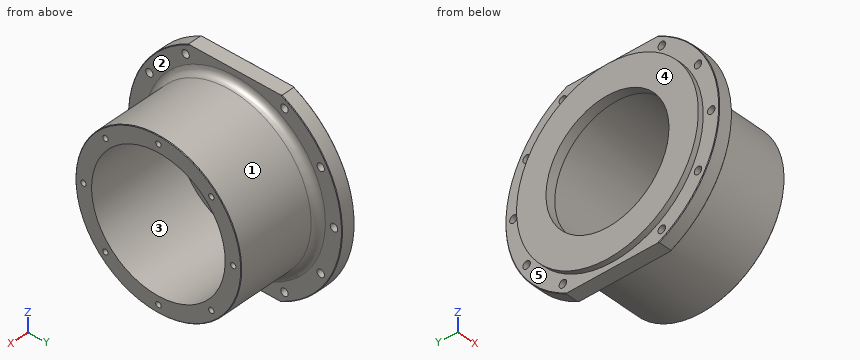
from build123d import *

# Parameters (mm, degrees)
CUT_EXTRUDE_1_REACH = 163.991
CUT_EXTRUDE_2_REACH = 164.985
SKETCH_5_R          = 3.5
SKETCH_6_R          = 2.5
CUT_EXTRUDE_3_DEPTH = 15
FILLET_1_R          = 7
CHAMFER_1_SIZE      = 0.5


with BuildPart() as part:
    # 草图1 → 旋转1 (revolve)
    with BuildSketch(Plane.XY, mode=Mode.PRIVATE) as revolve_1_sk:
        Polygon((0, 0), (0, 85), (5, 85), (5, 100), (18, 100), (18, 77.5), (97, 77.5), (97, 0), align=None)
    revolve(revolve_1_sk.sketch.rotate(Axis((0, 0, 0), (-1, 0, 0)), 90), axis=Axis((0, 0, 0), (-1, 0, 0)))

    # 草图3 → 切除-旋转1 (revolve, cut)
    with BuildSketch(Plane.XY, mode=Mode.PRIVATE) as cut_revolve_1_sk:
        Polygon((0, 0), (0, 57.5), (9, 57.5), (9, 62.5), (97, 62.5), (97, 0), align=None)
    revolve(cut_revolve_1_sk.sketch.rotate(Axis((97, 0, 0), (-1, 0, 0)), 90), axis=Axis((97, 0, 0), (-1, 0, 0)), mode=Mode.SUBTRACT)

    # 草图4 → 切除-拉伸1 (cut, up to next)
    with BuildSketch(Plane(origin=(18, 0, 0), x_dir=(0, 0, -1), z_dir=(1, 0, 0)), mode=Mode.PRIVATE) as cut_extrude_1_sk1:
        with BuildLine():
            Line((-90, 43.588989435), (-90, -43.588989435))
            ThreePointArc((-90, -43.588989435), (-100, 0), (-90, 43.588989435))
        make_face()
    cut_extrude_1_tool1 = extrude(cut_extrude_1_sk1.sketch, amount=-CUT_EXTRUDE_1_REACH, mode=Mode.PRIVATE) & part.part
    # 草图4 → 切除-拉伸1 (cut, up to next)
    with BuildSketch(Plane(origin=(18, 0, 0), x_dir=(0, 0, -1), z_dir=(1, 0, 0)), mode=Mode.PRIVATE) as cut_extrude_1_sk2:
        with BuildLine():
            Line((90, 43.588989435), (90, -43.588989435))
            ThreePointArc((90, -43.588989435), (100, 0), (90, 43.588989435))
        make_face()
    cut_extrude_1_tool2 = extrude(cut_extrude_1_sk2.sketch, amount=-CUT_EXTRUDE_1_REACH, mode=Mode.PRIVATE) & part.part
    add(cut_extrude_1_tool1.solids().sort_by_distance((18, 0, 94.017654))[0], mode=Mode.SUBTRACT)
    add(cut_extrude_1_tool2.solids().sort_by_distance((18, 0, -94.017654))[0], mode=Mode.SUBTRACT)

    # 草图5 → 切除-拉伸2 (cut, up to next)
    with BuildSketch(Plane.ZY.offset(-5), mode=Mode.PRIVATE) as cut_extrude_2_sk1:
        with Locations((0, 92.5)):
            Circle(SKETCH_5_R)
    cut_extrude_2_tool1 = extrude(cut_extrude_2_sk1.sketch, amount=-CUT_EXTRUDE_2_REACH, mode=Mode.PRIVATE) & part.part
    # 草图5 → 切除-拉伸2 (cut, up to next)
    with BuildSketch(Plane.ZY.offset(-5), mode=Mode.PRIVATE) as cut_extrude_2_sk2:
        with Locations((46.25, 80.10734985)):
            Circle(SKETCH_5_R)
    cut_extrude_2_tool2 = extrude(cut_extrude_2_sk2.sketch, amount=-CUT_EXTRUDE_2_REACH, mode=Mode.PRIVATE) & part.part
    # 草图5 → 切除-拉伸2 (cut, up to next)
    with BuildSketch(Plane.ZY.offset(-5), mode=Mode.PRIVATE) as cut_extrude_2_sk3:
        with Locations((80.10734985, 46.25)):
            Circle(SKETCH_5_R)
    cut_extrude_2_tool3 = extrude(cut_extrude_2_sk3.sketch, amount=-CUT_EXTRUDE_2_REACH, mode=Mode.PRIVATE) & part.part
    # 草图5 → 切除-拉伸2 (cut, up to next)
    with BuildSketch(Plane.ZY.offset(-5), mode=Mode.PRIVATE) as cut_extrude_2_sk4:
        with Locations((80.10734985, -46.25)):
            Circle(SKETCH_5_R)
    cut_extrude_2_tool4 = extrude(cut_extrude_2_sk4.sketch, amount=-CUT_EXTRUDE_2_REACH, mode=Mode.PRIVATE) & part.part
    # 草图5 → 切除-拉伸2 (cut, up to next)
    with BuildSketch(Plane.ZY.offset(-5), mode=Mode.PRIVATE) as cut_extrude_2_sk5:
        with Locations((46.25, -80.10734985)):
            Circle(SKETCH_5_R)
    cut_extrude_2_tool5 = extrude(cut_extrude_2_sk5.sketch, amount=-CUT_EXTRUDE_2_REACH, mode=Mode.PRIVATE) & part.part
    # 草图5 → 切除-拉伸2 (cut, up to next)
    with BuildSketch(Plane.ZY.offset(-5), mode=Mode.PRIVATE) as cut_extrude_2_sk6:
        with Locations((0, -92.5)):
            Circle(SKETCH_5_R)
    cut_extrude_2_tool6 = extrude(cut_extrude_2_sk6.sketch, amount=-CUT_EXTRUDE_2_REACH, mode=Mode.PRIVATE) & part.part
    # 草图5 → 切除-拉伸2 (cut, up to next)
    with BuildSketch(Plane.ZY.offset(-5), mode=Mode.PRIVATE) as cut_extrude_2_sk7:
        with Locations((-46.25, -80.10734985)):
            Circle(SKETCH_5_R)
    cut_extrude_2_tool7 = extrude(cut_extrude_2_sk7.sketch, amount=-CUT_EXTRUDE_2_REACH, mode=Mode.PRIVATE) & part.part
    # 草图5 → 切除-拉伸2 (cut, up to next)
    with BuildSketch(Plane.ZY.offset(-5), mode=Mode.PRIVATE) as cut_extrude_2_sk8:
        with Locations((-80.10734985, -46.25)):
            Circle(SKETCH_5_R)
    cut_extrude_2_tool8 = extrude(cut_extrude_2_sk8.sketch, amount=-CUT_EXTRUDE_2_REACH, mode=Mode.PRIVATE) & part.part
    # 草图5 → 切除-拉伸2 (cut, up to next)
    with BuildSketch(Plane.ZY.offset(-5), mode=Mode.PRIVATE) as cut_extrude_2_sk9:
        with Locations((-80.10734985, 46.25)):
            Circle(SKETCH_5_R)
    cut_extrude_2_tool9 = extrude(cut_extrude_2_sk9.sketch, amount=-CUT_EXTRUDE_2_REACH, mode=Mode.PRIVATE) & part.part
    # 草图5 → 切除-拉伸2 (cut, up to next)
    with BuildSketch(Plane.ZY.offset(-5), mode=Mode.PRIVATE) as cut_extrude_2_sk10:
        with Locations((-46.25, 80.10734985)):
            Circle(SKETCH_5_R)
    cut_extrude_2_tool10 = extrude(cut_extrude_2_sk10.sketch, amount=-CUT_EXTRUDE_2_REACH, mode=Mode.PRIVATE) & part.part
    add(cut_extrude_2_tool1.solids().sort_by_distance((5, 92.5, 0))[0], mode=Mode.SUBTRACT)
    add(cut_extrude_2_tool2.solids().sort_by_distance((5, 80.10735, 46.25))[0], mode=Mode.SUBTRACT)
    add(cut_extrude_2_tool3.solids().sort_by_distance((5, 46.25, 80.10735))[0], mode=Mode.SUBTRACT)
    add(cut_extrude_2_tool4.solids().sort_by_distance((5, -46.25, 80.10735))[0], mode=Mode.SUBTRACT)
    add(cut_extrude_2_tool5.solids().sort_by_distance((5, -80.10735, 46.25))[0], mode=Mode.SUBTRACT)
    add(cut_extrude_2_tool6.solids().sort_by_distance((5, -92.5, 0))[0], mode=Mode.SUBTRACT)
    add(cut_extrude_2_tool7.solids().sort_by_distance((5, -80.10735, -46.25))[0], mode=Mode.SUBTRACT)
    add(cut_extrude_2_tool8.solids().sort_by_distance((5, -46.25, -80.10735))[0], mode=Mode.SUBTRACT)
    add(cut_extrude_2_tool9.solids().sort_by_distance((5, 46.25, -80.10735))[0], mode=Mode.SUBTRACT)
    add(cut_extrude_2_tool10.solids().sort_by_distance((5, 80.10735, -46.25))[0], mode=Mode.SUBTRACT)

    # 草图6 → 切除-拉伸3 (cut)
    with BuildSketch(Plane(origin=(97, 0, 0), x_dir=(0, 0, -1), z_dir=(1, 0, 0))):
        with Locations((0, 70)):
            Circle(SKETCH_6_R)
        with Locations((49.497474683, 49.497474683)):
            Circle(SKETCH_6_R)
        with Locations((70, 0)):
            Circle(SKETCH_6_R)
        with Locations((49.497474683, -49.497474683)):
            Circle(SKETCH_6_R)
        with Locations((0, -70)):
            Circle(SKETCH_6_R)
        with Locations((-49.497474683, -49.497474683)):
            Circle(SKETCH_6_R)
        with Locations((-70, 0)):
            Circle(SKETCH_6_R)
        with Locations((-49.497474683, 49.497474683)):
            Circle(SKETCH_6_R)
    extrude(amount=-CUT_EXTRUDE_3_DEPTH, mode=Mode.SUBTRACT)

    # 圆角1
    fillet_1_edges = [part.edges().sort_by_distance(p)[0] for p in [
        (18, 0, 77.5),
    ]]
    fillet(fillet_1_edges, radius=FILLET_1_R)

    # 倒角1
    chamfer_1_edges = [part.edges().sort_by_distance(p)[0] for p in [
        (18, -100, 0),
        (5, -100, 0),
        (97, 0, 77.5),
        (18, 100, 0),
        (5, 100, 0),
    ]]
    chamfer(chamfer_1_edges, length=CHAMFER_1_SIZE)


solid = part.part
CAD build for the part. Positions are in the model's coordinates, mm. Face numbers are marked on the shaded views. A direction names the side the tool comes from. Coordinates: 2 decimals unless noted, no trailing zeros. Write each loop counter-clockwise with the first axis right and the second up, starting at its lowest first coordinate (ties: lowest second). Pieces come first, ordered by that corner, then holes. Notation, with made-up numbers: (-28, 29) - (-2, 29) arc R15 ccw to (-2, 49) - close; hole circle Ø11 at (-8.5, -13.5). An arc over 180 degrees is marked (long way). Use a Markdown table: item, result. Add a question column.
Item 1: Band-saw the part on B-B, the plane z = 0. Give the number of separate pieces and of enclosed holes in the cut face, and give its area (3 significant figures).
Item 2: Mould opens along Z. For the marked faces 1, 2 and 3 say: pulls with the +Z half, pulls with the -Z half, needs draft (parallel to the pull), parting line crosses it, or undercut.
Item 3: Band-saw the part on A-A, the plane x = 40.5. Give the cut face in (y, z).
Item 4: Drill centre lines: L1, parallel to Y at x = 14, z = 0; L2, parallel to Y at x = 90, z = 0; L3, parallel to Z at x = 10.5, y = -77. Where is each one in solid material? Low to high. Write a range as from..to.
Item 5: Flat gauge pins, fed straight in: pin 1 (4.5 mm diameter, centred on y = 49.5, z = 49.5, fed in from +X); pin 2 (1 mm diameter, centred on x = 26, z = 39.5, fed in from +Y); pin 3 (10 mm diameter, centred on x = 64.5, y = 34.5, fed in from -Z). Where does each tip first touch, or does it go through?
Item 6: 3-axis set-ups, long thin cutter, end or side, ignore diameter. For the marked faces 4 and 5: which of +Z, -Z, +X, -X, +Y, -Y reach the whole face in a straight line?
Numbers:
| question | item | result |
|---|---|---|
| 1 | separate pieces | 4 |
| 1 | enclosed holes | 0 |
| 1 | area | 3,350 mm2 |
| 2 | face 1 | parting line crosses it |
| 2 | face 2 | needs draft |
| 2 | face 3 | undercut |
| 3 | outline | circle Ø155 at (0, 0); hole circle Ø125 at (0, 0) |
| 4 | L1 | -100..-96, -89..-62.5, 62.5..89, 96..100 |
| 4 | L2 | -77.5..-72.5, -67.5..-62.5, 62.5..67.5, 72.5..77.5 |
| 4 | L3 | -63.8..-47.86, -44.64..44.64, 47.86..63.8 |
| 5 | pin 1 | x = 82 |
| 5 | pin 2 | y = 66.97 |
| 5 | pin 3 | z = -71.67 |
| 6 | face 4 | +Z, -Z, -X, +Y, -Y |
| 6 | face 5 | -X |
